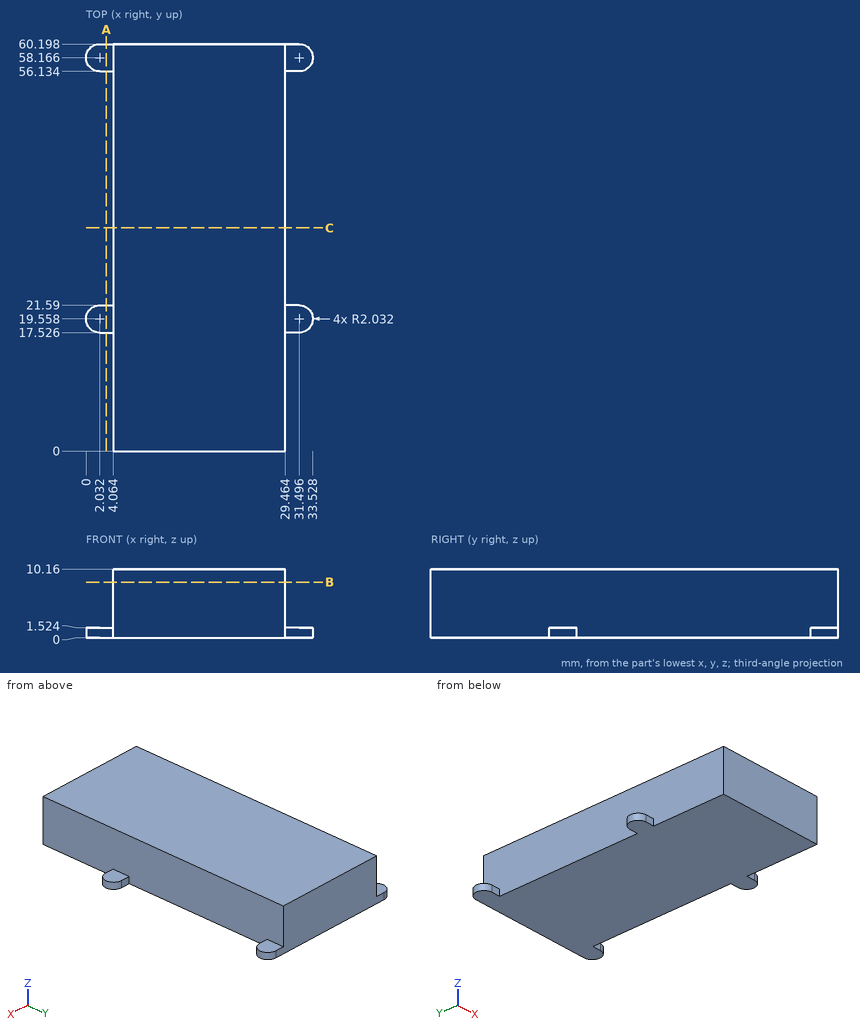
Geometry check sheet. Reference: drawing and pictorial views, mm from the part's lowest x, y, z. Give positions to 0.01 mm unless a question says otherwise; leave off trailing zeros. Order: outer loops, then holes, each group sorted by start corner. A loop starts at its lowest first (then second) coordinate and runs counter-clockwise, first axis right, second up. Notation, with made-up numbers: (-36, 27.5) - (5, 27.5) arc R33 ccw to (5, 57.5) - close; hole circle Ø3 at (-32.5, -4). An arc over 180 degrees is marked (long way). Use one line per item in the form item = value.
1) Depth check by flat-ended pin: pin 1 Ø1.7 at (x, z) = (2.5, 0.5) entering from -Y; pin 2 Ø5 at (y, z) = (29.5, 5) entering from -X; pin 3 Ø1.2 at (x, y) = (1.5, 19) entering from +Z. Enter the tip coordinate at first touch or a pass-through.
Working result:
pin_1 = 17.53
pin_2 = 4.06
pin_3 = 1.52
2) Sectioned sample at A-A (x = 3). Record the boundary of the cut face in (y, z).
Working result:
outline = (17.53, 0) - (21.59, 0) - (21.59, 1.52) - (17.53, 1.52) - close; (56.13, 0) - (60.2, 0) - (60.2, 1.52) - (56.13, 1.52) - close
3) Sectioned sample at C-C (y = 33). Record the boundary of the cut face in (x, z).
Working result:
outline = (4.06, 0) - (29.46, 0) - (29.46, 10.16) - (4.06, 10.16) - close
4) Material ranges on probe 1 along Y at (x, z) = (4, 1.25); probe 2 along X at (y, z) = (56, 9), recorded low to high. Write a range as from..to.
Working result:
probe_1 = 17.53..21.59, 56.13..60.2
probe_2 = 4.06..29.46
5) Sectioned sample at B-B (z = 8.25). Record the boundary of the cut face in (x, y), and give its area (3 significant figures).
Working result:
outline = (4.06, 0) - (29.46, 0) - (29.46, 60.2) - (4.06, 60.2) - close
area = 1,530 mm^2
